```python
from build123d import *

# Parameters (mm, degrees)
SKETCH018_W     = 16
SKETCH018_H     = 13.125
PAD006_DEPTH    = 1.6
SKETCH019_W     = 28.2
SKETCH019_H     = 13.125
PAD007_DEPTH    = 2
SKETCH020_R     = 1.7
POCKET007_DEPTH = 2


with BuildPart() as part:
    # Sketch018 → Pad006 (new body)
    with BuildSketch(Plane.XY):
        with Locations((0, 28.2)):
            Rectangle(SKETCH018_W, SKETCH018_H)
    extrude(amount=PAD006_DEPTH)

    # Sketch019 (on Face6 of Pad006) → Pad007 (join)
    with BuildSketch(Plane.XY.offset(1.6)):
        with Locations((0, 28.2)):
            Rectangle(SKETCH019_W, SKETCH019_H)
    extrude(amount=PAD007_DEPTH)

    # Sketch020 (on Face7 of Pad007) → Pocket007 (cut)
    with BuildSketch(Plane.XY.offset(3.6)):
        with Locations((-11.1, 28.7625)):
            Circle(SKETCH020_R)
        with Locations((11.1, 28.7625)):
            Circle(SKETCH020_R)
    extrude(amount=-POCKET007_DEPTH, mode=Mode.SUBTRACT)


with BuildPart() as part_1:
    # Body003 placement: moved
    add(part.part.moved(Location((0, 0, 2.4))))


solid = part_1.part
```
Work out the finished part from the listing and answer in its coordinate system (mm). A direction names the side the tool comes from. Coordinates: 2 decimals unless noted, no trailing zeros. Write each loop counter-clockwise with the first axis right and the second up, starting at its lowest first coordinate (ties: lowest second). Pieces come first, ordered by that corner, then holes.
Q1. Find the intervals of material crossed by line 1 (Y direction, x = -11.1, z = 5.35); line 2 (Z direction, x = -8.5, y = 28.75); line 3 (X direction, y = 24, z = 3.6), in increasing order.
Q2. Which of the six approach directions +Z, -Z, +X, -X, +Y, -Y give full straight-line access (tool end or side, diameter ignored) to faces 1 (the face through (8, 28, 3)), 2 (the face through (0, 21.638, 5)), 3 (the face through (-8, 28, 3))?
Q3. A cutting plane is placed at D-D, the plane y = 32.75. Give the vertices of the cut face in (x, z), then the cut area to 3 significant figures.
Q4. Each of these flat-tipped pins is pushed along its axis until it touches: pin 1 Ø1.8 at (x, y) = (-12.5, 29.5) entering from -Z; pin 2 Ø1.5 at (x, z) = (-11, 3) entering from -Y; pin 3 Ø0.8 at (y, z) = (29.5, 3.5) entering from -X; pin 4 Ø1.3 at (y, z) = (26.5, 3) entering from +X. Where does it stop, or does it pass through?
Q5. A cutting plane is placed at A-A, the plane x = -11.1. Give the vertices of the cut face in (y, z), then the cut area to 4 significant figures.
Q6. A cutting plane is placed at B-B, the plane y = 29.25. Give the vertices of the cut face in (x, z), then the cut area to 3 significant figures.
Q7. A cutting plane is placed at C-C, the plane z = 5.55. Give the vertices of the cut face in (x, y), then the cut area to 3 significant figures.
Q8. Determine the mould class of faces 4 (the face through (14.1, 28, 5)), 5 (the face through (12.01, 30.2, 5.01)), 6 (the face through (-11.1, 26.8, 4)) for opening direction X: released by +X, released by -X, zero draft, split by the parting line, or undercut.
Findings below:
1. line 1: y = 21.64 to 27.06, 30.46 to 34.76
1. line 2: z = 4 to 6
1. line 3: x = -8 to 8
2. face 1: -Z, +X, +Y, -Y
2. face 2: +Z, -Z, +X, -X, -Y
2. face 3: -Z, -X, +Y, -Y
3. outline: (-14.1, 4) - (-8, 4) - (-8, 2.4) - (8, 2.4) - (8, 4) - (14.1, 4) - (14.1, 6) - (-14.1, 6) - close
3. area: 82.0 mm2
4. pin 1: stops at z = 4
4. pin 2: passes through
4. pin 3: stops at x = -8
4. pin 4: stops at x = 8
5. outline: (21.64, 4) - (27.06, 4) - (27.06, 6) - (21.64, 6) - close; (30.46, 4) - (34.76, 4) - (34.76, 6) - (30.46, 6) - close
5. area: 19.45 mm2
6. outline: (-14.1, 4) - (-12.73, 4) - (-12.73, 6) - (-14.1, 6) - close; (-9.47, 4) - (-8, 4) - (-8, 2.4) - (8, 2.4) - (8, 4) - (9.47, 4) - (9.47, 6) - (-9.47, 6) - close; (12.73, 4) - (14.1, 4) - (14.1, 6) - (12.73, 6) - close
6. area: 69.0 mm2
7. outline: (-14.1, 21.64) - (14.1, 21.64) - (14.1, 34.76) - (-14.1, 34.76) - close; hole circle Ø3.4 at (-11.1, 28.76); hole circle Ø3.4 at (11.1, 28.76)
7. area: 352 mm2
8. face 4: released by +X
8. face 5: undercut
8. face 6: zero draft
